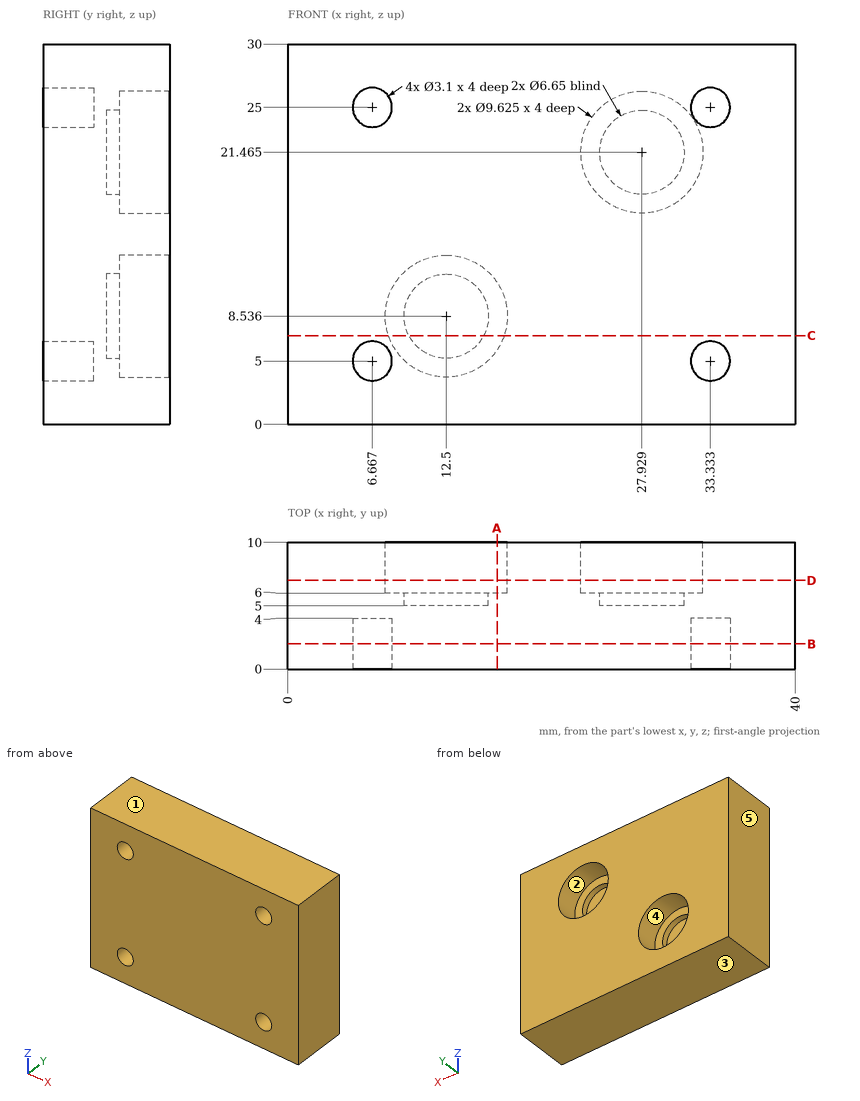
Input: dimensioned drawing with shaded views. Units: mm. Origin: part minimum x, y, z. A direction names the side the tool comes from. Round coordinates to 2 decimals unless told otherwise and drop trailing zeros. Loops run counter-clockwise (first coordinate to the right, second up) from the corner with the lowest first, then second, coordinate; pieces in that order, holes last. Notation, with made-up numbers: M -14.5,27.5 L -9.5,27.5 A21 ccw -9.5,60.5 Z; hole C 5,67 d9. An arc over 180 degrees is marked long. Return JSON: item names as keys, results as strings. Group by question number.
1. Pin query (flat end, axial travel): pin 1 (5.5 mm diameter, centred on x = 12.5, z = 8.54, fed in from +Y); pin 2 (5 mm diameter, centred on x = 13, z = 9.5, fed in from +Y); pin 3 (0.9 mm diameter, centred on x = 33.5, z = 25.5, fed in from -Y). Return the tip coordinate at first contact, or that it passes through.
2. Section query B-B on y = 2. Output: boundary loops of the cut face in (x, z).
3. Section query C-C on z = 7. Output: boundary loops of the cut face in (x, y), and give its area (3 significant figures).
4. Reachability of the marked faces 4 and 5 from +Z, -Z, +X, -X, +Y, -Y: full face, straight path, thin tool, end or side. Return the list, or none.
5. Material intervals for line 1 along X through (y, z) = (9.5, 8.25); line 2 along Z through (x, y) = (32, 2.25); line 3 along Z through (x, y) = (31, 7.5), sorted ascending. Write a range as from..to.
6. Mould query, pull axis Z, two halves, no side actions, for the marked faces 1, 2 and 3. Classes: released by +Z, released by -Z, zero draft, split by the parting line, or undercut.
7. Section query D-D on y = 7. Output: boundary loops of the cut face in (x, z) (1 decimal).
8. Section query A-A on x = 16.5. Output: boundary loops of the cut face in (y, z).
Checks:
{
 "1": {"pin 1": "stops at y = 5", "pin 2": "stops at y = 6", "pin 3": "stops at y = 4"},
 "2": {"outline": "M 0,0 L 40,0 L 40,30 L 0,30 Z; hole C 6.67,5 d3.1; hole C 6.67,25 d3.1; hole C 33.33,5 d3.1; hole C 33.33,25 d3.1"},
 "3": {"outline": "M 0,0 L 40,0 L 40,10 L 17.06,10 L 17.06,6 L 15.45,6 L 15.45,5 L 9.55,5 L 9.55,6 L 7.94,6 L 7.94,10 L 0,10 Z", "area": "358 mm²"},
 "4": {"face 4": "+Y", "face 5": "+Z, -Z, -X, +Y, -Y"},
 "5": {"line 1": "x = 0..7.7, 17.3..40", "line 2": "z = 0..4.21, 5.79..24.21, 25.79..30", "line 3": "z = 0..17.76, 25.17..30"},
 "6": {"face 1": "released by +Z", "face 2": "undercut", "face 3": "released by -Z"},
 "7": {"outline": "M 0,0 L 40,0 L 40,30 L 0,30 Z; hole C 12.5,8.5 d9.6; hole C 27.9,21.5 d9.6"},
 "8": {"outline": "M 0,0 L 10,0 L 10,5.86 L 6,5.86 L 6,11.21 L 10,11.21 L 10,30 L 0,30 Z"}
}
